from build123d import *

# Parameters (mm, degrees)
SKETCH1_W               = 50
SKETCH1_H               = 50
BOSS_EXTRUDE1_DEPTH     = 100
SKETCH4_R               = 2.5
BOSS_EXTRUDE2_DEPTH     = 4.5
CUT_EXTRUDE1_DEPTH      = 161.078105936
CUT_EXTRUDE1_DEPTH_BACK = 161.078105936
SKETCH5_R               = 2.5
SKETCH6_W               = 50
SKETCH6_H               = 50
CUT_EXTRUDE2_DEPTH      = 4.5
CUT_EXTRUDE5_DEPTH      = 161.078105936
CUT_EXTRUDE5_DEPTH_BACK = 161.078105936
CHAMFER1_SIZE           = 12


with BuildPart() as part:
    # Sketch1 → Boss-Extrude1 (new body)
    with BuildSketch(Plane(origin=(0, 0, 0), x_dir=(1, 0, 0), z_dir=(0, 1, 0))):
        Rectangle(SKETCH1_W, SKETCH1_H)
    extrude(amount=BOSS_EXTRUDE1_DEPTH)

    # Sketch4 → Boss-Extrude2 (add)
    with BuildSketch(Plane(origin=(0, 0, -25), x_dir=(-1, 0, 0), z_dir=(0, 0, -1))):
        with BuildLine():
            Line((-25, 100), (25, 100))
            Line((25, 100), (25, 125))
            ThreePointArc((25, 125), (0, 150), (-25, 125))
            Line((-25, 125), (-25, 100))
        make_face()
        with Locations((0, 125)):
            Circle(SKETCH4_R, mode=Mode.SUBTRACT)
    boss_extrude2 = extrude(amount=-BOSS_EXTRUDE2_DEPTH)

    # Mirror2: Boss-Extrude2 across plane
    add(boss_extrude2.mirror(Plane.XY))

    # Sketch5 → Cut-Extrude1 (cut, two sides: drawn at the far end of the back side and taken through both)
    with BuildSketch(Plane.ZY.offset(-25).offset(-CUT_EXTRUDE1_DEPTH_BACK)):
        with BuildLine():
            Line((-25, 0), (2.6e-08, 0))
            ThreePointArc((2.6e-08, 0), (-17.67766952, 7.322330461), (-25, 25))
            Line((-25, 25), (-25, 0))
        make_face()
        with BuildLine():
            Line((25, 0), (25, 25))
            ThreePointArc((25, 25), (17.677669539, 7.32233048), (2.6e-08, 0))
            Line((2.6e-08, 0), (25, 0))
        make_face()
        with Locations((0, 25)):
            Circle(SKETCH5_R)
    extrude(amount=CUT_EXTRUDE1_DEPTH + CUT_EXTRUDE1_DEPTH_BACK, mode=Mode.SUBTRACT)

    # Sketch6 → Cut-Extrude2 (cut)
    with BuildSketch(Plane(origin=(25, 0, 0), x_dir=(0, 0, -1), z_dir=(1, 0, 0))):
        with Locations((0, 25)):
            Rectangle(SKETCH6_W, SKETCH6_H)
    cut_extrude2 = extrude(amount=-CUT_EXTRUDE2_DEPTH, mode=Mode.SUBTRACT)

    # Mirror3: Cut-Extrude2 across plane
    add(cut_extrude2.mirror(Plane(origin=(0, 0, 0), x_dir=(0, 0, 1), z_dir=(1, 0, 0))), mode=Mode.SUBTRACT)

    # Sketch8 → Cut-Extrude5 (cut, two sides: drawn at the far end of the back side and taken through both)
    with BuildSketch(Plane(origin=(25, 0, 0), x_dir=(0, 0, -1), z_dir=(1, 0, 0)).offset(-CUT_EXTRUDE5_DEPTH_BACK)):
        Polygon((-25, 80), (-3.250930707, 32.404472018), (11.086507283, 32.404472018), (25, 80), (47.596959839, 33.904901575), (18.755369464, -23.278135991), (-42.095384797, 0), align=None)
    extrude(amount=CUT_EXTRUDE5_DEPTH + CUT_EXTRUDE5_DEPTH_BACK, mode=Mode.SUBTRACT)

    # Chamfer1
    chamfer1_edges = [part.edges().sort_by_distance(p)[0] for p in [
        (25, 65, 18.145657728),
        (-25, 65, 18.145657728),
    ]]
    chamfer(chamfer1_edges, length=CHAMFER1_SIZE)

    # Chamfer2
    # the kernel refuses this chamfer: 15 mm, written as the material it takes off along each edge
    with BuildSketch(Plane(origin=(25, -38.861557394, 9.746529416), x_dir=(0.02749587661058632, 0.2804786274156753, 0.9594663706104734), z_dir=(0, 0.9598292658239239, -0.2805847117501368)), Plane(origin=(-25, 168.861557394, -50.976697476), x_dir=(-0.027495876610586306, 0.2804786274156753, 0.9594663706104732), z_dir=(0, -0.9598292658239239, 0.2805847117501368))) as chamfer2_piece_1:
        with BuildLine():
            Line((15.430097928, 0), (-0.848207323, -15.406766903))
            Line((-0.848207323, -15.406766903), (-1.148093898, -15.39851814))
            ThreePointArc((-1.148093898, -15.39851814), (-0.511938406, -7.700967445), (-0.299886575, 0.008248763))
            Line((-0.299886575, 0.008248763), (0.008248763, 0.299886575))
            ThreePointArc((0.008248763, 0.299886575), (7.717464971, 0.087834744), (15.438346691, 0.299886575))
            Line((15.438346691, 0.299886575), (15.430097928, 0))
        make_face()
    extrude(amount=216.416733875, mode=Mode.SUBTRACT)


solid = part.part
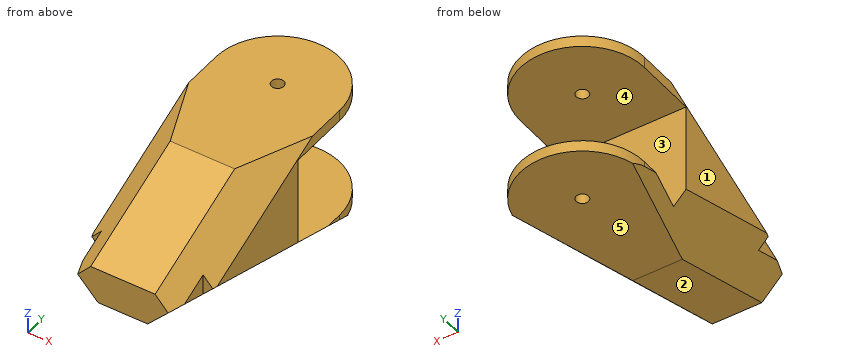
Can you work these out from the model? Positions are in its coordinate system, mm. Face numbers are marked on the shaded views. A direction names the side the tool comes from. Coordinates: 2 decimals unless noted, no trailing zeros. Loops run counter-clockwise (first coordinate to the right, second up) from the corner with the lowest first, then second, coordinate; pieces in that order, holes last. Notation, with made-up numbers: (-14, -4) - (21, -4) arc R16 ccw to (21, 8) - close; hole circle Ø2 at (38.5, 31). An arc over 180 degrees is marked (long way). Answer as a JSON object with one key per item and string values. Group by question number.
Item 1: If we section it at D-D (y = 84.5): List the corners of the cut face in (x, z) for me.
Item 2: On a 3-axis mill with a long thin cutter (end or side, diameter ignored), from which of +Z, -Z, +X, -X, +Y, -Y can I reach the whole of each face in a straight line? I mean the marked faces 4 and 5. Say none if no direction works.
Item 3: If we mould it in two halves opening along Z, with no side actions, what happens to the marked faces 1, 2 and 3? For each: released by +Z, released by -Z, zero draft, split by the parting line, or undercut.
Item 4: If I drill on L1, parallel to Y at x = 13.5, z = -6.5; L2, parallel to Z at x = 3, y = 143; L3, parallel to Y at x = 0, z = 22, over which ranges is the centre line in solid material (lowest first)? Write a range as from..to.
Item 5: For pin 1 (10 mm diameter, centred on y = 62.5, z = -18, fed in from -X); pin 2 (1.9 mm diameter, centred on x = 21.5, z = 1, fed in from -Y); pin 3 (1.5 mm diameter, centred on x = -6, z = -13.5, fed in from +Y); pin 4 (3 mm diameter, centred on x = 0, y = 125, fed in from -Z), each with a flat end and sliding along its axis, tell me the tip position at first contact or that it passes through.
Item 6: If we section it at A-A (x = 0): List the corners of the cut face in (y, z) for me.
Item 7: If we section it at C-C (x = -8.5): List the corners of the cut face in (y, z) for me, plus the area to 3 significant figures.
Item 8: If we section it at B-B (y = 136.5): List the corners of the cut face in (x, z) for me, plus the area to 3 significant figures.
Returned:
{
 "1": {"outline": "(-25, -10.69) - (-11.26, -25) - (11.26, -25) - (25, -10.69) - (25, 13.86) - (14.87, 25) - (-14.87, 25) - (-25, 13.86) - close"},
 "2": {"face 4": "+X, -X, +Y", "face 5": "-Z, +X, -X, +Y, -Y"},
 "3": {"face 1": "zero draft", "face 2": "released by -Z", "face 3": "undercut"},
 "4": {"L1": "y = 32.4..100", "L2": "z = -25..-20.5, 20.5..25", "L3": "y = 73.43..122.5, 127.5..150"},
 "5": {"pin 1": "stops at x = -16.81", "pin 2": "stops at y = 50", "pin 3": "stops at y = 100", "pin 4": "passes through"},
 "6": {"outline": "(32.4, -11.09) - (80, -25) - (122.5, -25) - (122.5, -20.5) - (100, -20.5) - (100, 20.5) - (122.5, 20.5) - (122.5, 25) - (80, 25) - (32.4, 3.25) - close; (127.5, -25) - (150, -25) - (150, -20.5) - (127.5, -20.5) - close; (127.5, 20.5) - (150, 20.5) - (150, 25) - (127.5, 25) - close"},
 "7": {"outline": "(32.4, -11.09) - (80, -25) - (148.51, -25) - (148.51, -20.5) - (100, -20.5) - (100, 20.5) - (148.51, 20.5) - (148.51, 25) - (80, 25) - (32.4, 3.25) - close", "area": "2,970 mm²"},
 "8": {"outline": "(-22.2, -25) - (22.2, -25) - (22.2, -20.5) - (-22.2, -20.5) - close; (-22.2, 20.5) - (22.2, 20.5) - (22.2, 25) - (-22.2, 25) - close", "area": "400 mm²"}
}
